Autodesk Inventor part; units mm, degrees
ref_plane "YZ Plane" through (0, 0, 0) normal (1, 0, 0) x (0, 1, 0)
ref_plane "XZ Plane" through (0, 0, 0) normal (0, 1, 0) x (-1, 0, 0)
ref_plane "XY Plane" through (0, 0, 0) normal (0, 0, 1) x (1, 0, 0)
sketch "Эскиз1" plane through (0, 0, 0) normal (0, 0, 1) x (1, 0, 0)
  line L0 (130, 0) -> (130, 4)
  line L1 (140, 4) -> (130, 4)
  line L2 (140, 0) -> (140, 4)
  line L3 (140, 0) -> (130, 0)
  line L4 (120, 0) -> (120, 4)
  line L5 (120, 4) -> (110, 4)
  line L6 (110, 4) -> (110, 0)
  line L7 (120, 0) -> (110, 0)
  line L8 (90, 4) -> (90, 0)
  line L9 (100, 0) -> (90, 0)
  line L10 (100, 0) -> (100, 4)
  line L11 (100, 4) -> (90, 4)
  line L12 (80, 0) -> (80, 4)
  line L13 (80, 4) -> (70, 4)
  line L14 (70, 4) -> (70, 0)
  line L15 (80, 0) -> (70, 0)
  line L16 (50, 4) -> (50, 0)
  line L17 (60, 0) -> (50, 0)
  line L18 (60, 0) -> (60, 4)
  line L19 (60, 4) -> (50, 4)
  line L20 (40, 0) -> (40, 4)
  line L21 (40, 4) -> (30, 4)
  line L22 (30, 4) -> (30, 0)
  line L23 (40, 0) -> (30, 0)
  line L24 (10, 4) -> (10, 0)
  line L25 (20, 0) -> (10, 0)
  line L26 (20, 0) -> (20, 4)
  line L27 (20, 4) -> (10, 4)
  line L28 (0, 0) -> (0, 4)
  line L29 (0, 4) -> (-10, 4)
  line L30 (-10, 4) -> (-10, 0)
  line L31 (0, 0) -> (-10, 0)
  line L32 (-20, 4) -> (-10, 4)
  line L33 (-20, 4) -> (140, 4)
  line L34 (-20, 4) -> (-20, 104)
  line L35 (140, 4) -> (176.397, 104)
  line L36 (140, 4) -> (246.4178, 4) construction
  line L37 (176.397, 104) -> (-20, 104)
  line L38 (-20, 94) -> (-16, 94)
  line L39 (-16, 94) -> (-16, 84)
  line L40 (-16, 84) -> (-20, 84)
  line L41 (-20, 84) -> (-20, 94)
  line L42 (-16, 74) -> (-16, 64)
  line L43 (-20, 64) -> (-20, 74)
  line L44 (-20, 74) -> (-16, 74)
  line L45 (-16, 64) -> (-20, 64)
  line L46 (-16, 54) -> (-16, 44)
  line L47 (-20, 44) -> (-20, 54)
  line L48 (-20, 54) -> (-16, 54)
  line L49 (-16, 44) -> (-20, 44)
  line L50 (-16, 34) -> (-16, 24)
  line L51 (-20, 24) -> (-20, 34)
  line L52 (-20, 34) -> (-16, 34)
  line L53 (-16, 24) -> (-20, 24)
  line L54 (-16, 14) -> (-16, 4)
  line L55 (-20, 4) -> (-20, 14)
  line L56 (-20, 14) -> (-16, 14)
  line L57 (-16, 4) -> (-20, 4)
  line L58 (172.7573, 94) -> (169.3371, 84.6031)
  line L59 (169.3371, 84.6031) -> (165.5783, 85.9712)
  line L60 (165.5783, 85.9712) -> (168.9986, 95.3681)
  line L61 (168.9986, 95.3681) -> (172.7573, 94)
  line L62 (158.7379, 67.1773) -> (162.1581, 76.5742)
  line L63 (165.9169, 75.2061) -> (162.4967, 65.8092)
  line L64 (162.1581, 76.5742) -> (165.9169, 75.2061)
  line L65 (162.4967, 65.8092) -> (158.7379, 67.1773)
  line L66 (151.8975, 48.3834) -> (155.3177, 57.7804)
  line L67 (159.0765, 56.4123) -> (155.6563, 47.0154)
  line L68 (155.3177, 57.7804) -> (159.0765, 56.4123)
  line L69 (155.6563, 47.0154) -> (151.8975, 48.3834)
  line L70 (145.0571, 29.5896) -> (148.4773, 38.9865)
  line L71 (152.2361, 37.6184) -> (148.8159, 28.2215)
  line L72 (148.4773, 38.9865) -> (152.2361, 37.6184)
  line L73 (148.8159, 28.2215) -> (145.0571, 29.5896)
  line L74 (138.2167, 10.7957) -> (141.6369, 20.1927)
  line L75 (145.3957, 18.8246) -> (141.9755, 9.4277)
  line L76 (141.6369, 20.1927) -> (145.3957, 18.8246)
  line L77 (141.9755, 9.4277) -> (138.2167, 10.7957)
  dimension "d0" = 100
  dimension "d1" = 70
  dimension "d2" = 4
  dimension "d3" = 10
  dimension "d4" = 10
  dimension "d7" = 20
  dimension "d12" = 10
  dimension "d13" = 4
  dimension "d14" = 10
  dimension "d17" = 20
extrude "Выдавливание1" add sketch "Эскиз1" along normal blind 4 contours L0 L1 L2 L3 | L33 L5 L11 L13 L19 L21 L27 L29 L32 L54 L56 L34 L53 L50 L52 L49 L46 L48 L45 L42 L44 L40 L39 L38 L37 L35 L61 L60 L59 L64 L62 L65 L68 L66 L69 L72 L70 L73 L76 L74 L77 L1 | L4 L7 L6 L5 | L10 L9 L8 L11 | L12 L15 L14 L13 | L18 L17 L16 L19 | L20 L23 L22 L21 | L26 L25 L24 L27 | L28 L31 L30 L29
sketch "Эскиз2" plane through (0, 0, 0) normal (0, 0, -1) x (-1, 0, 0)
  line L0 (-172.7573, 94) -> (-176.397, 104)
  line L1 (16, 4) -> (-176.397, 104) construction
  line L2 (-176.397, 104) -> (-140, 0)
  line L3 (-140, 0) -> (20, 104) construction
  line L4 (-68.0944, 4) -> (-68.0944, 104) construction
  line L5 (-176.397, 104) -> (20, 104)
  circle A0 centre (-68.0944, 54) radius 7
  line L6 (-60, 4) -> (-70, 4)
  point P0 (0, 0)
  dimension "d24" = 100
  dimension "d25" = 14
  dimension "d26" = 50
extrude "Выдавливание2" cut sketch "Эскиз2" against normal blind 10
sketch "Эскиз3" plane through (0, 0, 4) normal (0, 0, 1) x (1, 0, 0)
  circle A0 centre (68.0944, 54) radius 7
  circle A1 centre (68.0944, 54) radius 6.25
  circle A2 centre (59.0944, 63) radius 4
  circle A3 centre (59.0944, 45) radius 4
  circle A4 centre (92.0944, 63) radius 3.5
  circle A5 centre (92.0944, 63) radius 4
  circle A6 centre (92.0944, 45) radius 4
  circle A7 centre (80.5944, 48) radius 3.5
  circle A8 centre (80.5944, 60) radius 3.5
  circle A9 centre (68.0944, 54) radius 6.75
  point P0 (0, 0)
extrude "Выдавливание3" cut sketch "Эскиз3" against normal blind 10 contours A0 | A1 | A2 | A3 | A4 | A5 | A6 | A7 | A8 | A9
properties part number "боковушка"
Work out the finished part from the listing and answer in its coordinate system (mm). A direction names the side the tool comes from. Give positions to 0.01 mm unless a question says otherwise; leave off trailing zeros. Return JSON: item names as keys, results as strings.
1) A tool of negligible diameter and unlimited length cuts with its end or side. For faces 1 (the flat face through (0, 2, 2)), 2 (the flat face through (-13, 4, 2)), 3 (the flat face through (-18, 94, 2)), 4 (the flat face through (140.122, 10.102, 1.972)), 5 (the flat face through (-20, 99, 2)), from which of +Z, -Z, +X, -X, +Y, -Y can it reach the whole face along a straight path? Write none if from no direction.
Resolved:
{"face 1": "+Z, -Z, -Y", "face 2": "+Z, -Z, -X, -Y", "face 3": "+Z, -Z, -X", "face 4": "+Z, -Z, +X", "face 5": "+Z, -Z, -X, +Y, -Y"}
2) Straight lines are drawn through the part: line 1 along Y through (x, z) = (92, 2.2); line 2 along X through (y, z) = (58.5, 2.2); line 3 along Y through (x, z) = (72, 1.6). For each, find the intervals that lie inside material, in ascending order. Write a range as [from, to].
Resolved:
{"line 1": "[0, 41], [49, 59], [67, 104]", "line 2": "[-20, 62.73], [73.46, 77.43], [83.76, 159.84]", "line 3": "[0, 48.19], [59.81, 104]"}
3) For a pull along Y with two mould halves and no side action, classify faces 6 (the flat face through (80, 104, 2)), 7 (the flat face through (-16, 89, 2)), 8 (the flat face through (10, 2, 2)) as +Y half, -Y half, draft (parallel to the pull), parting line (faces both ways), or undercut.
Resolved:
{"face 6": "+Y half", "face 7": "undercut", "face 8": "draft"}
4) Section A-A, the plane z = 0.75 is taken. Give the number of separate pieces and of enclosed holes in the cut face, plus the area to 3 significant figures.
Resolved:
{"separate pieces": "1", "enclosed holes": "7", "area": "17,300 mm^2"}
5) Each of these flat-tipped pins is pushed along its axis until it touches: pin 1 (2 mm diameter, centred on x = -18.5, z = 2.5, fed in from -Y); pin 2 (2 mm diameter, centred on y = 1.5, z = 2, fed in from +X); pin 3 (1 mm diameter, centred on y = 31.5, z = 1.5, fed in from -X). Where does it stop, or does it pass through?
Resolved:
{"pin 1": "y = 14", "pin 2": "x = 140", "pin 3": "x = -16"}
